```python
from build123d import *

# Parameters (mm, degrees)
SKETCH_1_W          = 80
SKETCH_1_H          = 52
EXTRUDE_1_DEPTH     = 5
CUT_EXTRUDE_3_DEPTH = 10
CUT_EXTRUDE_4_DEPTH = 10
SKETCH_9_R          = 1
CUT_EXTRUDE_5_DEPTH = 10
SKETCH_10_W         = 5
SKETCH_10_H         = 5
CUT_EXTRUDE_6_DEPTH = 10
SKETCH_11_R         = 1
CUT_EXTRUDE_7_DEPTH = 10
SKETCH_12_W         = 5
SKETCH_12_H         = 9.9
EXTRUDE_4_DEPTH     = 5
SKETCH_13_R         = 1
CUT_EXTRUDE_8_DEPTH = 5
FILLET_2_R          = 2
SKETCH_14_W         = 14
SKETCH_14_H         = 5
EXTRUDE_5_DEPTH     = 5
FILLET_3_R          = 1


with BuildPart() as part:
    # 스케치1 → 보스-돌출1 (new body)
    with BuildSketch(Plane.XY):
        with Locations((-10, -8.537755654)):
            Rectangle(SKETCH_1_W, SKETCH_1_H)
    extrude(amount=EXTRUDE_1_DEPTH)

    # 스케치7 → 컷-돌출3 (cut)
    with BuildSketch(Plane(origin=(0, 0, 0), x_dir=(-1, 0, 0), z_dir=(0, 0, -1))):
        with BuildLine():
            Line((-30, 2.012244346), (-24, 2.012244346))
            Line((-24, 2.012244346), (-24, 3.212244346))
            ThreePointArc((-24, 3.212244346), (-22.6, 4.612244346), (-21.2, 3.212244346))
            Line((-21.2, 3.212244346), (-21.2, 2.012244346))
            Line((-21.2, 2.012244346), (-20, 2.012244346))
            ThreePointArc((-20, 2.012244346), (-18.45, 0.462244346), (-20, -1.087755654))
            Line((-20, -1.087755654), (-21.2, -1.087755654))
            Line((-21.2, -1.087755654), (-21.2, -2.287755654))
            ThreePointArc((-21.2, -2.287755654), (-22.6, -3.687755654), (-24, -2.287755654))
            Line((-24, -2.287755654), (-24, -1.087755654))
            Line((-24, -1.087755654), (-30, -1.087755654))
            Line((-30, -1.087755654), (-30, 2.012244346))
        make_face()
        with BuildLine():
            Line((-30, -22.987755654), (-24, -22.987755654))
            Line((-24, -22.987755654), (-24, -21.787755654))
            ThreePointArc((-24, -21.787755654), (-22.6, -20.387755654), (-21.2, -21.787755654))
            Line((-21.2, -21.787755654), (-21.2, -22.987755654))
            Line((-21.2, -22.987755654), (-20, -22.987755654))
            ThreePointArc((-20, -22.987755654), (-18.45, -24.537755654), (-20, -26.087755654))
            Line((-20, -26.087755654), (-21.2, -26.087755654))
            Line((-21.2, -26.087755654), (-21.2, -27.287755654))
            ThreePointArc((-21.2, -27.287755654), (-22.6, -28.687755654), (-24, -27.287755654))
            Line((-24, -27.287755654), (-24, -26.087755654))
            Line((-24, -26.087755654), (-30, -26.087755654))
            Line((-30, -26.087755654), (-30, -22.987755654))
        make_face()
        with BuildLine():
            Line((44, -27.287755654), (44, -26.087755654))
            Line((44, -26.087755654), (50, -26.087755654))
            Line((50, -26.087755654), (50, -22.987755654))
            Line((50, -22.987755654), (44, -22.987755654))
            Line((44, -22.987755654), (44, -21.787755654))
            ThreePointArc((44, -21.787755654), (42.6, -20.387755654), (41.2, -21.787755654))
            Line((41.2, -21.787755654), (41.2, -22.987755654))
            Line((41.2, -22.987755654), (40, -22.987755654))
            ThreePointArc((40, -22.987755654), (38.45, -24.537755654), (40, -26.087755654))
            Line((40, -26.087755654), (41.2, -26.087755654))
            Line((41.2, -26.087755654), (41.2, -27.287755654))
            ThreePointArc((41.2, -27.287755654), (42.6, -28.687755654), (44, -27.287755654))
        make_face()
        with BuildLine():
            Line((44, -2.287755654), (44, -1.087755654))
            Line((44, -1.087755654), (50, -1.087755654))
            Line((50, -1.087755654), (50, 2.012244346))
            Line((50, 2.012244346), (44, 2.012244346))
            Line((44, 2.012244346), (44, 3.212244346))
            ThreePointArc((44, 3.212244346), (42.6, 4.612244346), (41.2, 3.212244346))
            Line((41.2, 3.212244346), (41.2, 2.012244346))
            Line((41.2, 2.012244346), (40, 2.012244346))
            ThreePointArc((40, 2.012244346), (38.45, 0.462244346), (40, -1.087755654))
            Line((40, -1.087755654), (41.2, -1.087755654))
            Line((41.2, -1.087755654), (41.2, -2.287755654))
            ThreePointArc((41.2, -2.287755654), (42.6, -3.687755654), (44, -2.287755654))
        make_face()
    extrude(amount=-CUT_EXTRUDE_3_DEPTH, mode=Mode.SUBTRACT)

    # 스케치8 → 컷-돌출4 (cut)
    with BuildSketch(Plane(origin=(0, 0, 0), x_dir=(-1, 0, 0), z_dir=(0, 0, -1))):
        with BuildLine():
            Line((19.200961894, 9.398777825), (21.799038106, 7.898777825))
            ThreePointArc((21.799038106, 7.898777825), (29.485571585, -20.787755654), (0.799038106, -28.474289134))
            Line((0.799038106, -28.474289134), (-1.799038106, -26.974289134))
            ThreePointArc((-1.799038106, -26.974289134), (-9.485571585, 1.712244346), (19.200961894, 9.398777825))
        make_face()
    extrude(amount=-CUT_EXTRUDE_4_DEPTH, mode=Mode.SUBTRACT)

    # 스케치9 → 컷-돌출5 (cut)
    with BuildSketch(Plane(origin=(0, 0, 0), x_dir=(-1, 0, 0), z_dir=(0, 0, -1))):
        with Locations((-14.248711306, 4.462244346)):
            Circle(SKETCH_9_R)
    extrude(amount=-CUT_EXTRUDE_5_DEPTH, mode=Mode.SUBTRACT)

    # 스케치10 → 컷-돌출6 (cut)
    with BuildSketch(Plane.XY.offset(5)):
        with Locations((13.5, -32.037755654)):
            Rectangle(SKETCH_10_W, SKETCH_10_H)
        with Locations((-33.5, -32.037755654)):
            Rectangle(SKETCH_10_W, SKETCH_10_H)
    extrude(amount=-CUT_EXTRUDE_6_DEPTH, mode=Mode.SUBTRACT)

    # 스케치11 → 컷-돌출7 (cut)
    with BuildSketch(Plane(origin=(0, 0, 0), x_dir=(-1, 0, 0), z_dir=(0, 0, -1))):
        with Locations((-11, -30.537755654)):
            Circle(SKETCH_11_R)
        with Locations((-16, -30.537755654)):
            Circle(SKETCH_11_R)
        with Locations((31, -30.537755654)):
            Circle(SKETCH_11_R)
        with Locations((36, -30.537755654)):
            Circle(SKETCH_11_R)
    extrude(amount=-CUT_EXTRUDE_7_DEPTH, mode=Mode.SUBTRACT)

    # 스케치12 → 보스-돌출4 (add)
    with BuildSketch(Plane(origin=(0, 0, 0), x_dir=(-1, 0, 0), z_dir=(0, 0, -1))):
        with Locations((52.5, -12.037755654)):
            Rectangle(SKETCH_12_W, SKETCH_12_H)
        with Locations((-32.5, -12.037755654)):
            Rectangle(SKETCH_12_W, SKETCH_12_H)
    extrude(amount=-EXTRUDE_4_DEPTH)

    # 스케치13 → 컷-돌출8 (cut)
    with BuildSketch(Plane(origin=(0, 0, 0), x_dir=(-1, 0, 0), z_dir=(0, 0, -1))):
        with Locations((50, -6.087755654)):
            Circle(SKETCH_13_R)
        with Locations((50, -17.987755654)):
            Circle(SKETCH_13_R)
        with Locations((-30, -6.087755654)):
            Circle(SKETCH_13_R)
        with Locations((-30, -17.987755654)):
            Circle(SKETCH_13_R)
    extrude(amount=-CUT_EXTRUDE_8_DEPTH, mode=Mode.SUBTRACT)

    # 필렛2
    fillet_2_edges = [part.edges().sort_by_distance(p)[0] for p in [
        (-55, -7.087755654, 2.5),
        (-55, -16.987755654, 2.5),
        (35, -7.087755654, 2.5),
        (35, -16.987755654, 2.5),
    ]]
    fillet(fillet_2_edges, radius=FILLET_2_R)

    # 스케치14 → 보스-돌출5 (add)
    with BuildSketch(Plane(origin=(0, 0, 0), x_dir=(-1, 0, 0), z_dir=(0, 0, -1))):
        with Locations((43, -37.037755654)):
            Rectangle(SKETCH_14_W, SKETCH_14_H)
        with Locations((-23, -37.037755654)):
            Rectangle(SKETCH_14_W, SKETCH_14_H)
    extrude(amount=-EXTRUDE_5_DEPTH)

    # 필렛3
    fillet_3_edges = [part.edges().sort_by_distance(p)[0] for p in [
        (-50, -39.537755654, 2.5),
        (-36, -39.537755654, 2.5),
        (16, -39.537755654, 2.5),
        (30, -39.537755654, 2.5),
    ]]
    fillet(fillet_3_edges, radius=FILLET_3_R)


solid = part.part
```
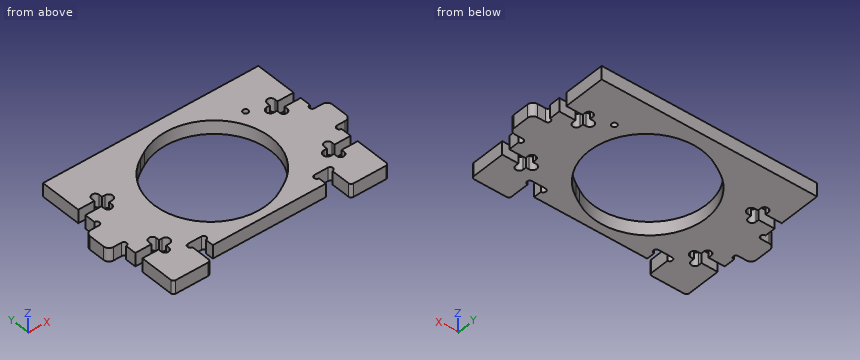
Here's how the part is built. I have some questions about the finished solid (model axes, mm). Coordinates: 2 decimals unless noted, no trailing zeros. Order: outer loops, then holes, each group sorted by start corner. A loop starts at its lowest first (then second) coordinate and runs counter-clockwise, first axis right, second up. Notation, with made-up numbers: M 32,9.5 L 40,9.5 A15 cw 40,28.5 Z; hole C 13,-30 d7. An arc over 180 degrees is marked long. Answer as a JSON object with one key per item and string values. Group by question number.
(1) Suppose I cut it at B-B, the plane x = 22.6. Please give me the cut outline in (y, z).
(2) Suppose I cut it at D-D, the plane y = -12. Please give me the cut outline in (x, z), then the cut area to 3 significant figures.
(3) Suppose I cut it at A-A, the plane y = -33. Please give me the cut outline in (x, z).
(4) Suppose I cut it at C-C, the plane x = -10.5. Please give me the cut outline in (y, z), then the cut area to 3 significant figures.
(5) For pin 1 (1 mm diameter, centred on y = -26.5, z = 2, fed in from -X); pin 2 (0.6 mm diameter, centred on y = -1.5, z = 2.5, fed in from +X); pin 3 (2.5 mm diameter, centred on x = 32, z = 2, fed in from -Y), each with a flat end and sliding along its axis, tell me the tip position at first contact or that it passes through.
(6) I need wall thicknesses on probe 1 along Y at (x, z) = (-47.5, 4.5); probe 2 along X at (y, z) = (-32.5, 2.3); probe 3 along X at (y, z) = (-37, 0.35). Which ranges of each line are inside material? Lowest first, please.
Values found:
{
 "1": {"outline": "M -39.54,0 L -28.69,0 L -28.69,5 L -39.54,5 Z; M -20.39,0 L -3.69,0 L -3.69,5 L -20.39,5 Z; M 4.61,0 L 17.46,0 L 17.46,5 L 4.61,5 Z"},
 "2": {"outline": "M -55,0 L -32.23,0 L -32.23,5 L -55,5 Z; M 12.05,0 L 35,0 L 35,5 L 12.05,5 Z", "area": "229 mm^2"},
 "3": {"outline": "M -50,0 L -36,0 L -36,5 L -50,5 Z; M -31,0 L 11,0 L 11,5 L -31,5 Z; M 16,0 L 30,0 L 30,5 L 16,5 Z"},
 "4": {"outline": "M -34.54,0 L -31.27,0 L -31.27,5 L -34.54,5 Z; M 12.14,0 L 17.46,0 L 17.46,5 L 12.14,5 Z", "area": "43.0 mm^2"},
 "5": {"pin 1": "stops at x = -50", "pin 2": "stops at x = 30", "pin 3": "stops at y = -16.99"},
 "6": {"probe 1": "y = -39.54 to -26.09, -22.99 to -1.09, 2.01 to 17.46", "probe 2": "x = -50 to -36, -31 to 11, 16 to 30", "probe 3": "x = -50 to -36, 16 to 30"}
}
